from build123d import *

# Parameters (mm, degrees)
F2_R = 1.5
F3_R = 0.5


with BuildPart() as f1:
    # F0 (on Front) → F1 (revolve)
    with BuildSketch(Plane.XZ):
        Polygon((0, 16.5), (0, 13), (6.25, 13), (6.25, 6), (20, 6), (20, 0), (22.5, 0), (22.5, 8.5), (9.25, 8.5), (9.25, 16.5), align=None)
    revolve(axis=Axis((0, 0, 14.75), (0, 0, 1)))

    # F2
    f2_edges = [f1.edges().sort_by_distance(p)[0] for p in [
        (-9.25, 0, 8.5),
    ]]
    fillet(f2_edges, radius=F2_R)

    # F3
    f3_edges = [f1.edges().sort_by_distance(p)[0] for p in [
        (-22.5, 0, 8.5),
    ]]
    fillet(f3_edges, radius=F3_R)


solid = f1.part
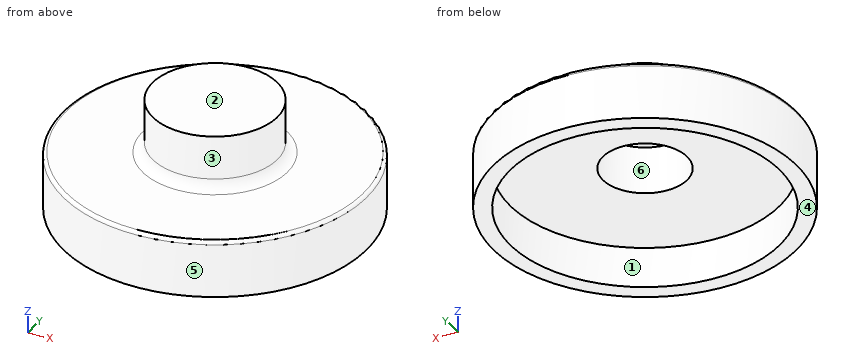
Geometry: final body of the model. Coordinates: model frame, mm. Face numbers are marked on the shaded views. A direction names the side the tool comes from. Give positions to 0.01 mm unless a question says otherwise; leave off trailing zeros. Loops run counter-clockwise (first coordinate to the right, second up) from the corner with the lowest first, then second, coordinate; pieces in that order, holes last. Notation, with made-up numbers: M -18.75,4.5 L -14.75,4.5 A26 cw -14.75,29.5 Z; hole C 79,5.25 d6. An arc over 180 degrees is marked long. Put each result on its own line as item: value. Start each with the question number.
1) Cut plane C-C (z = 3.5). Output: boundary loops of the cut face in (x, y).
2) Pull-direction query (X, two-part tool) for the marked faces 4, 5 and 6; classes: pulls with the +X half, pulls with the -X half, needs draft (parallel to the pull), parting line crosses it, or undercut.
3) Ray query, line 1 along Y through (x, z) = (0, 2.1); line 2 along Y through (x, z) = (0, 11.25); line 3 along Z through (x, y) = (14, -11.5). Return the intervals inside material, ascending.
4) Cut plane A-A (y = 0). Output: boundary loops of the cut face in (x, z), then the cut area to 3 significant figures.
5) Contact query for flat-ended pins moving along their axis: pin 1 (1 mm diameter, centred on x = -6.5, y = 4, fed in from -Z); pin 2 (2 mm diameter, centred on x = -11.5, z = 5.5, fed in from -Y); pin 3 (4 mm diameter, centred on y = -4, z = 12.5, fed in from +X). Output: stop coordinate, or through.
6) Access query for the marked faces 1, 2 and 3. Directions: +Z, -Z, +X, -X, +Y, -Y. A direction counts if a zero-diameter tool reaches every point of the face in a straight line with its end or side. Return the directions, or none.
Verdict:
1. outline: C 0,0 d45; hole C 0,0 d40
2. face 4: needs draft
2. face 5: parting line crosses it
2. face 6: undercut
3. line 1: -22.5 to -20, 20 to 22.5
3. line 2: -9.25 to -6.25, 6.25 to 9.25
3. line 3: 6 to 8.5
4. outline: M -22.5,0 L -20,0 L -20,6 L -6.25,6 L -6.25,13 L 6.25,13 L 6.25,6 L 20,6 L 20,0 L 22.5,0 L 22.5,8 A0.5 ccw 22,8.5 L 10.75,8.5 A1.5 cw 9.25,10 L 9.25,16.5 L -9.25,16.5 L -9.25,10 A1.5 cw -10.75,8.5 L -22,8.5 A0.5 ccw -22.5,8 Z
4. area: 204 mm2
5. pin 1: z = 6
5. pin 2: y = -19.9
5. pin 3: x = 9.03
6. face 1: -Z
6. face 2: +Z, +X, -X, +Y, -Y
6. face 3: +Z
